Could you check a few things on this drawing? It's one solid part, dimensions in mm from its lowest x, y, z. A direction names the side the tool comes from. Coordinates: 2 decimals unless noted, no trailing zeros. Write each loop counter-clockwise with the first axis right and the second up, starting at its lowest first coordinate (ties: lowest second). Pieces come first, ordered by that corner, then holes. Notation, with made-up numbers: (22.5, 62) - (78.5, 62) arc R28 cw to (78.5, 85) - close; hole circle Ø5 at (-39, 3.25). An arc over 180 degrees is marked (long way). Answer as a JSON object with one key per item and string values. Group by question number.
1) Will these pins go through, and if not, where does the flat tip stop? pin 1 Ø2 at (x, y) = (30.5, 25.5) entering from +Z; pin 2 Ø5 at (x, y) = (18, 18) entering from +Z; pin 3 Ø6 at (x, z) = (32, 2.5) entering from -Y; pin 4 Ø5 at (x, z) = (28.5, 7.5) entering from +Y.
2) We'd pull the mould along X, two halves only. Please class the marked faces 1, 2 and 3: released by +X, released by -X, zero draft, split by the parting line, or undercut.
3) On a 3-axis mill with a long thin cutter (end or side, diameter ignored), from which of +Z, -Z, +X, -X, +Y, -Y can I reach the whole of each face in a straight line? I mean the marked faces 4 and 5. Say none if no direction works.
4) If we section it at D-D (z = 1): Write out the boundary of the cut face in (x, y), plus the area to 3 significant figures.
5) Please list where these lines run through material, in increasing order: line 1 along Y through (x, z) = (18, 7.5); line 2 along Y through (x, z) = (18, 1.85); line 3 along X through (y, z) = (4, 5).
6) If we section it at C-C (z = 8.25): Write out the boundary of the cut face in (x, y), plus the area to 3 significant figures.
7) If we section it at A-A (x = 18): Write out the boundary of the cut face in (y, z).
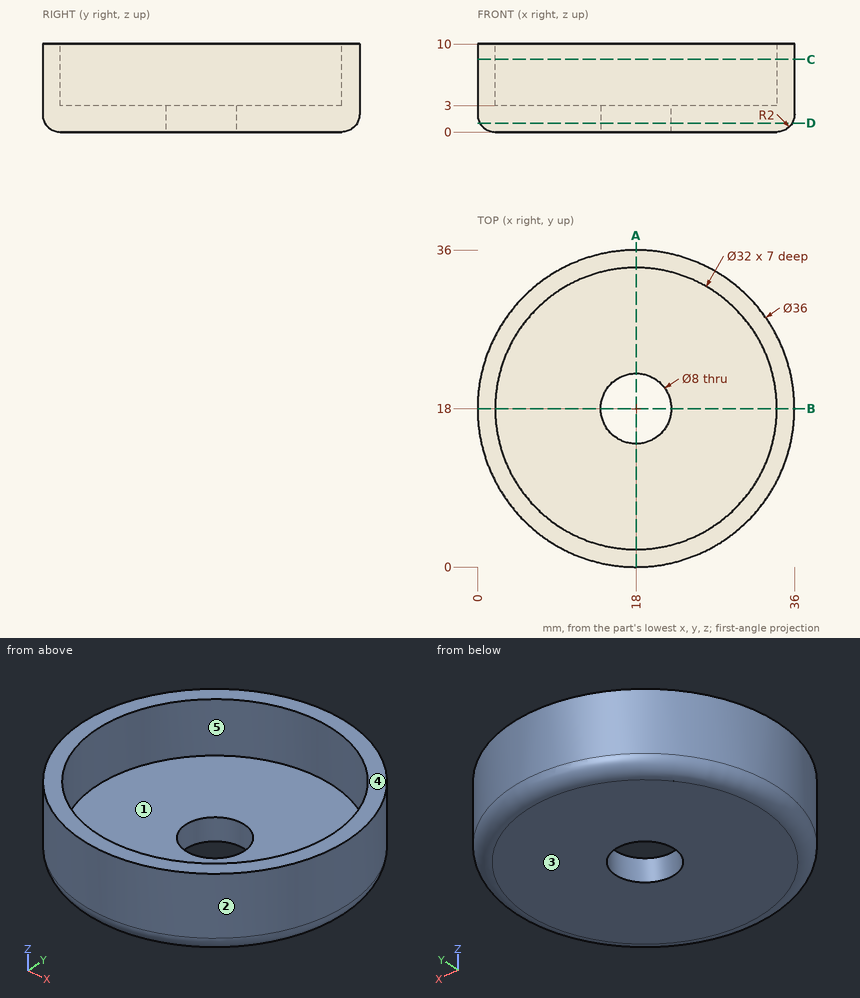
Here are the results:
{
 "1": {"pin 1": "stops at z = 3", "pin 2": "passes through", "pin 3": "stops at y = 3.75", "pin 4": "stops at y = 34.12"},
 "2": {"face 1": "undercut", "face 2": "split by the parting line", "face 3": "zero draft"},
 "3": {"face 4": "+Z, +X, -X, +Y, -Y", "face 5": "+Z"},
 "4": {"outline": "circle Ø35.46 at (18, 18); hole circle Ø8 at (18, 18)", "area": "938 mm²"},
 "5": {"line 1": "y = 0 to 2, 34 to 36", "line 2": "y = 0.01 to 14, 22 to 35.99", "line 3": "x = 6.69 to 10.25, 25.75 to 29.31"},
 "6": {"outline": "circle Ø36 at (18, 18); hole circle Ø32 at (18, 18)", "area": "214 mm²"},
 "7": {"outline": "(0, 2) arc R2 ccw to (2, 0) - (14, 0) - (14, 3) - (2, 3) - (2, 10) - (0, 10) - close; (22, 0) - (34, 0) arc R2 ccw to (36, 2) - (36, 10) - (34, 10) - (34, 3) - (22, 3) - close"}
}
